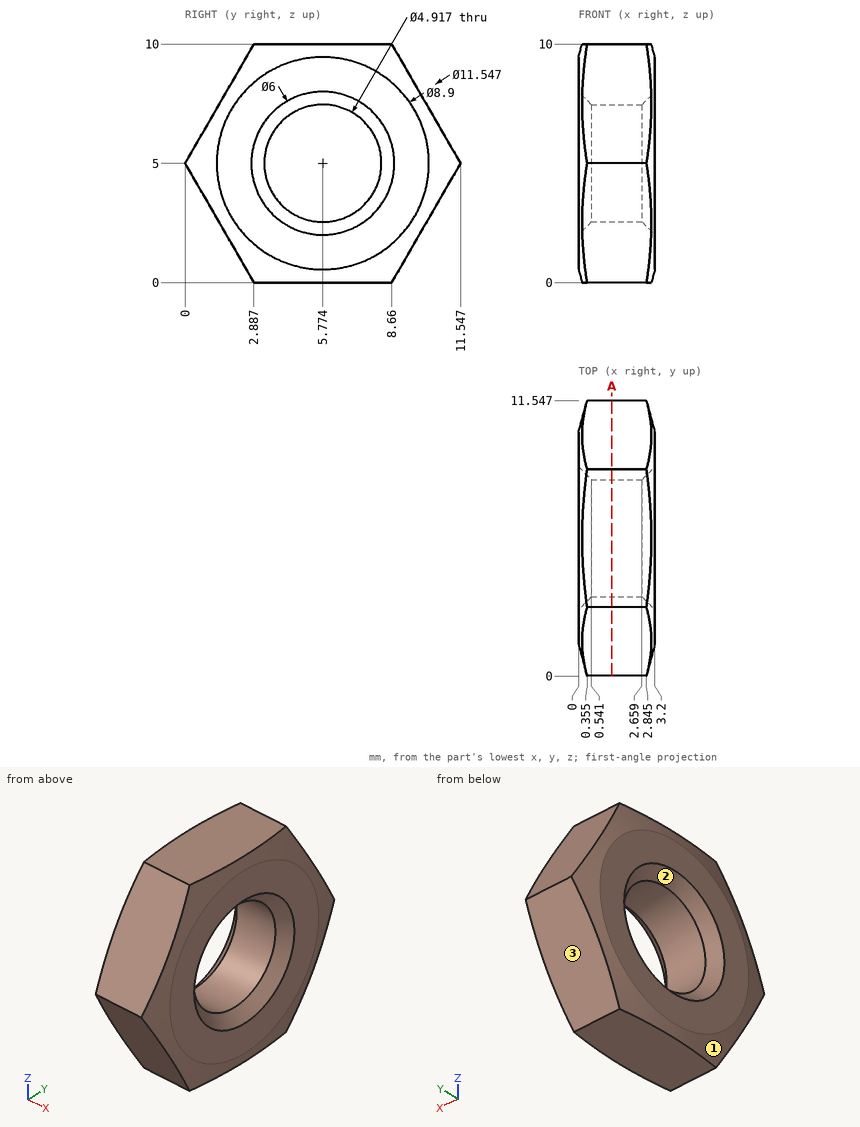
Answer from the drawing. Dimensions are ordinates in mm from the lowest x, y and z of the part. Give positions to 0.01 mm unless a question says otherwise; leave off trailing zeros. Write each loop counter-clockwise with the first axis right and the second up, starting at its lowest first coordinate (ties: lowest second). Pieces come first, ordered by that corner, then holes. Notation, with made-up numbers: (-16.5, 58) -> (20.5, 58) arc R26 ccw to (20.5, 92) -> close; hole circle Ø1 at (42.5, 62). An arc over 180 degrees is marked (long way). Use a Markdown table: item, result.
(1) Section A-A, the plane x = 1.4 is taken. Determine the outline of the cut face in (y, z).
Return value:
| item | result |
|---|---|
| outline | (0, 5) -> (2.89, 0) -> (8.66, 0) -> (11.55, 5) -> (8.66, 10) -> (2.89, 10) -> close; hole circle Ø4.92 at (5.77, 5) |
(2) Flat-ended cylindrical pins translate along their axes: P1, Ø1.5, axis at x = 0.5, z = 7.5, coming from the -Y side; P2, Ø5.5, axis at y = 5.77, z = 5, coming from the -X side (1 decimal). Find the tip coordinate at first contact, or state that the pin passes through.
Return value:
| item | result |
|---|---|
| P1 | y = 1.01 |
| P2 | x = 0.2 |
(3) Determine the mould class of the marked faces 1, 2 and 3 for opening direction Z: released by +Z, released by -Z, zero draft, split by the parting line, or undercut.
Return value:
| item | result |
|---|---|
| face 1 | split by the parting line |
| face 2 | undercut |
| face 3 | released by -Z |
(4) Find the intervals of material crossed by probe 1 along Z at (x, y) = (1.5, 5.75); probe 2 along Y at (x, z) = (0.7, 3.5) (1 decimal); probe 3 along Y at (x, z) = (0.2, 7.5) (1 decimal), in increasing order. Write a range as from..to.
Return value:
| item | result |
|---|---|
| probe 1 | 0..2.54, 7.46..10 |
| probe 2 | 0.9..3.8, 7.7..10.7 |
| probe 3 | 1.4..4.5, 7..10.1 |
